from build123d import *

# Parameters (mm, degrees)
CROQUIS1_W                   = 100
CROQUIS1_H                   = 60
CROQUIS1_R                   = 20
SALIENTE_EXTRUIR1_DEPTH      = 3
CROQUIS2_W                   = 10
CROQUIS2_H                   = 1
SALIENTE_EXTRUIR2_DEPTH      = 10
SALIENTE_EXTRUIR2_DEPTH_BACK = 3
CROQUIS3_R                   = 2.5
CORTAR_EXTRUIR1_DEPTH        = 1


with BuildPart() as part:
    # Croquis1 → Saliente-Extruir1 (new body)
    with BuildSketch(Plane(origin=(0, 0, 0), x_dir=(1, 0, 0), z_dir=(0, 1, 0))):
        Rectangle(CROQUIS1_W, CROQUIS1_H)
        Circle(CROQUIS1_R, mode=Mode.SUBTRACT)
    extrude(amount=SALIENTE_EXTRUIR1_DEPTH)

    # Croquis2 → Saliente-Extruir2 (add, two sides)
    with BuildSketch(Plane(origin=(0, 3, 0), x_dir=(1, 0, 0), z_dir=(0, 1, 0))) as saliente_extruir2_sk:
        with Locations((-20, 1.75)):
            Rectangle(CROQUIS2_W, CROQUIS2_H)
        with Locations((-20, -1.75)):
            Rectangle(CROQUIS2_W, CROQUIS2_H)
    extrude(amount=SALIENTE_EXTRUIR2_DEPTH)
    extrude(saliente_extruir2_sk.sketch, amount=-SALIENTE_EXTRUIR2_DEPTH_BACK)

    # Croquis3 → Cortar-Extruir1 (cut)
    with BuildSketch(Plane(origin=(0, 3, 0), x_dir=(1, 0, 0), z_dir=(0, 1, 0))):
        with Locations((25, 0)):
            Circle(CROQUIS3_R)
    extrude(amount=-CORTAR_EXTRUIR1_DEPTH, mode=Mode.SUBTRACT)


solid = part.part
The listing builds one solid part. Answer for the finished solid, in the listing's coordinates (mm). A direction names the side the tool comes from. Round coordinates to 2 decimals unless told otherwise and drop trailing zeros. Order: outer loops, then holes, each group sorted by start corner. A loop starts at its lowest first (then second) coordinate and runs counter-clockwise, first axis right, second up. Notation, with made-up numbers: M -14,40.25 L 37,40.25 A14 cw 37,46.25 Z; hole C 9,-6 d2. An arc over 180 degrees is marked long. Answer in a Markdown table with one row per item. Add a question column.
1) Consider line 1 along X through (y, z) = (2.85, 0); line 2 along Z through (x, y) = (25, 2.5); line 3 along X through (y, z) = (2.75, 9). Determine where each line is inside the solid, lowest interval first. Write a range as from..to.
2) The part is cut by section B-B on y = 4.25. Determine the outline of the cut face in (x, z).
3) Flat-ended cylindrical pins translate along their axes: pin 1 Ø3 at (x, y) = (-21, 7) entering from -Z; pin 2 Ø5 at (x, y) = (-20.5, 9.5) entering from +Z; pin 3 Ø1.1 at (y, z) = (6, -2) entering from -X. Find the tip coordinate at first contact, or state that the pin passes through.
4) The part is cut by section A-A on x = 0. Determine the outline of the cut face in (y, z).
5) The part is cut by section D-D on x = -28.5. Determine the outline of the cut face in (y, z), plus the area to 3 significant figures.
6) Which of the six approach directions +Z, -Z, +X, -X, +Y, -Y give full straight-line access (tool end or side, diameter ignored) to faces 5 (the face through (22.5, 2.5, -0.1)), 6 (the face through (-1, 1, -30))?
7) The part is cut by section C-C on x = 25. Determine the outline of the cut face in (y, z).
8) Determine the mould class of faces 1 (the face through (-50, 1, 0)), 2 (the face through (-20, 1, 0)), 3 (the face through (-20, 7, -1.25)), 4 (the face through (-1, 1, 30)) for opening direction Z: pulls with the +Z half, pulls with the -Z half, needs draft (parallel to the pull), parting line crosses it, or undercut.
Findings below:
| question | item | result |
|---|---|---|
| 1 | line 1 | x = -50..-20, 20..22.5, 27.5..50 |
| 1 | line 2 | z = -30..-2.5, 2.5..30 |
| 1 | line 3 | x = -50..-17.86, 17.86..50 |
| 2 | outline | M -25,-2.25 L -15,-2.25 L -15,-1.25 L -25,-1.25 Z; M -25,1.25 L -15,1.25 L -15,2.25 L -25,2.25 Z |
| 3 | pin 1 | stops at z = -2.25 |
| 3 | pin 2 | stops at z = 2.25 |
| 3 | pin 3 | stops at x = -25 |
| 4 | outline | M 0,-30 L 3,-30 L 3,-20 L 0,-20 Z; M 0,20 L 3,20 L 3,30 L 0,30 Z |
| 5 | outline | M 0,-30 L 3,-30 L 3,30 L 0,30 Z |
| 5 | area | 180 mm² |
| 6 | face 5 | +Y |
| 6 | face 6 | -Z, +X, -X, +Y, -Y |
| 7 | outline | M 0,-30 L 3,-30 L 3,-2.5 L 2,-2.5 L 2,2.5 L 3,2.5 L 3,30 L 0,30 Z |
| 8 | face 1 | needs draft |
| 8 | face 2 | undercut |
| 8 | face 3 | undercut |
| 8 | face 4 | pulls with the +Z half |
